from build123d import *

# Parameters (mm, degrees)
SKETCH2_R           = 47.5
SKETCH2_R_2         = 5
BOSS_EXTRUDE2_DEPTH = 26
CUT_EXTRUDE1_DEPTH  = 26


with BuildPart() as part:
    # Sketch2 → Boss-Extrude2 (new body)
    with BuildSketch(Plane.XY):
        with BuildLine():
            Line((-44.361418341, 36.582981874), (25.749824557, 121.601589362))
            ThreePointArc((25.749824557, 121.601589362), (35.699764064, 124.986391522), (43.181062365, 117.604768557))
            Line((43.181062365, 117.604768557), (70.382008245, 5.874854744))
            ThreePointArc((70.382008245, 5.874854744), (71.516417726, -3.340902868), (70.495441136, -12.569915818))
            Line((70.495441136, -12.569915818), (43.209420588, -130.966785703))
            ThreePointArc((43.209420588, -130.966785703), (35.417472002, -138.528541499), (25.323491774, -134.527769491))
            Line((25.323491774, -134.527769491), (-46.812831844, -33.388752219))
            ThreePointArc((-46.812831844, -33.388752219), (-57.464744559, 2.013239383), (-44.361418341, 36.582981874))
        make_face()
        with Locations(Location((0, 0, 0), (0, 0, 180))):
            Circle(SKETCH2_R, mode=Mode.SUBTRACT)
        with Locations(Location((33.464853834, 115.239331644, 0), (0, 0, 180))):
            Circle(SKETCH2_R_2, mode=Mode.SUBTRACT)
        with Locations(Location((33.464853834, -128.721029975, 0), (0, 0, 180))):
            Circle(SKETCH2_R_2, mode=Mode.SUBTRACT)
    extrude(amount=BOSS_EXTRUDE2_DEPTH)

    # Sketch3 → Cut-Extrude1 (cut)
    with BuildSketch(Plane(origin=(0, 0, 0), x_dir=(-1, 0, 0), z_dir=(0, 0, -1))):
        with BuildLine():
            Line((-33.26004361, 92.533263855), (-44.920341747, 51.273747369))
            ThreePointArc((-44.920341747, 51.273747369), (-44.16321834, 48.345074539), (-41.240708097, 47.564501493))
            Line((-41.240708097, 47.564501493), (2.410664417, 59.523781634))
            ThreePointArc((2.410664417, 59.523781634), (4.534059271, 61.712628945), (3.644196413, 64.629476961))
            Line((3.644196413, 64.629476961), (-28.346877964, 93.929713306))
            ThreePointArc((-28.346877964, 93.929713306), (-31.193307402, 94.603096407), (-33.26004361, 92.533263855))
        make_face()
        with BuildLine():
            Line((-41.486917876, -55.239236277), (2.503698589, -65.483626413))
            ThreePointArc((2.503698589, -65.483626413), (4.700165382, -67.55485567), (3.983155181, -70.48749158))
            Line((3.983155181, -70.48749158), (-28.256543188, -103.932412317))
            ThreePointArc((-28.256543188, -103.932412317), (-31.16488904, -104.755498955), (-33.313463379, -102.629569624))
            Line((-33.313463379, -102.629569624), (-45.064381475, -58.940258751))
            ThreePointArc((-45.064381475, -58.940258751), (-44.32436227, -56.076046257), (-41.486917876, -55.239236277))
        make_face()
    extrude(amount=-CUT_EXTRUDE1_DEPTH, mode=Mode.SUBTRACT)


solid = part.part
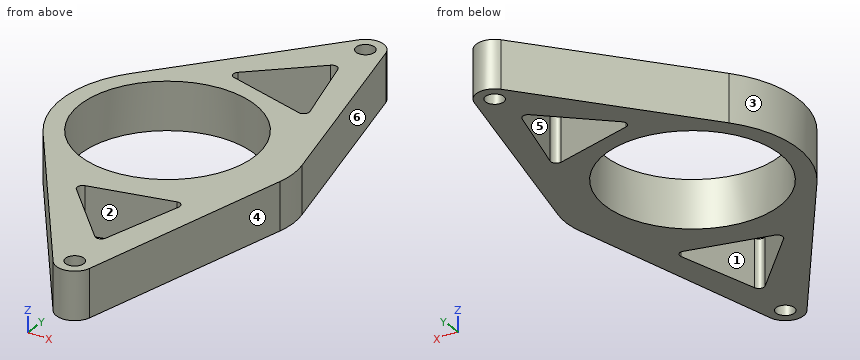
The listing builds one solid part. Answer for the finished solid, in the listing's coordinates (mm). Face numbers are marked on the shaded views. A direction names the side the tool comes from. Give positions to 0.01 mm unless a question says otherwise; leave off trailing zeros. Loops run counter-clockwise (first coordinate to the right, second up) from the corner with the lowest first, then second, coordinate; pieces in that order, holes last.
Item 1: Find the intervals of material crossed by line 1 along Y through (x, z) = (29, 19.5); line 2 along Y through (x, z) = (11, 24.75); line 3 along X through (y, z) = (88.5, 16), in increasing order.
Derived:
line 1: y = -137.67 to -130.97, -126.47 to -104.49, -58.15 to -37.62, 37.62 to 50.92, 94.38 to 112.99, 117.49 to 124.19
line 2: y = -114.45 to -86.03, -62.34 to -46.21, 46.21 to 55.85, 78.04 to 103.72
line 3: x = -1.55 to 22.42, 34.4 to 50.27
Item 2: Each of these flat-tipped pins is pushed along its axis until it touches: pin 1 Ø1 at (y, z) = (18.5, 18) entering from +X; pin 2 Ø8 at (y, z) = (-8, 12) entering from -X; pin 3 Ø2 at (x, z) = (-11.5, 20) entering from -Y. Where does it stop, or does it pass through?
Derived:
pin 1: stops at x = 67.43
pin 2: stops at x = -57.36
pin 3: stops at y = -84.3
Item 3: A cutting plane is placed at A-A (x = 12). Give the vertices of the cut face in (y, z), then the cut area to 3 significant figures.
Derived:
outline: (-115.85, 0) - (-87.07, 0) - (-87.07, 26) - (-115.85, 26) - close; (-62.11, 0) - (-45.96, 0) - (-45.96, 26) - (-62.11, 26) - close; (45.96, 0) - (55.58, 0) - (55.58, 26) - (45.96, 26) - close; (78.96, 0) - (104.93, 0) - (104.93, 26) - (78.96, 26) - close
area: 2,090 mm2
Item 4: Determine the mould class of the marked faces 1, 2, 3 and 4 for opening direction X: +X half, -X half, draft (parallel to the pull), parting line (faces both ways), or undercut.
Derived:
face 1: undercut
face 2: undercut
face 3: -X half
face 4: +X half
Item 5: A tool of negligible diameter and unlimited length cuts with its end or side. For the marked faces 5 and 6, from which of +Z, -Z, +X, -X, +Y, -Y can it reach the whole face along a straight path? Write none if from no direction.
Derived:
face 5: +Z, -Z
face 6: +Z, -Z, +X, +Y
Item 6: A cutting plane is placed at B-B (y = 90). Give the vertices of the cut face in (x, z), then the cut area to 3 significant figures.
Derived:
outline: (-0.31, 0) - (24.06, 0) - (24.06, 26) - (-0.31, 26) - close; (33.98, 0) - (49.9, 0) - (49.9, 26) - (33.98, 26) - close
area: 1,050 mm2
Item 7: A cutting plane is placed at C-C (x = -32). Give the vertices of the cut face in (y, z), then the cut area to 3 significant figures.
Derived:
outline: (-54.16, 0) - (-35.1, 0) - (-35.1, 26) - (-54.16, 26) - close; (35.1, 0) - (51.57, 0) - (51.57, 26) - (35.1, 26) - close
area: 924 mm2
Item 8: A cutting plane is placed at D-D (z = 19.5). Give the vertices of the cut face in (x, y), then the cut area to 3 significant figures.
Derived:
outline: (-46.81, -33.39) - (25.32, -134.53) arc R10 ccw to (43.21, -130.97) - (70.5, -12.57) arc R40 ccw to (70.38, 5.87) - (43.18, 117.6) arc R10 ccw to (25.75, 121.6) - (-44.36, 36.58) arc R57.5 ccw to start; hole circle Ø95 at (0, 0); hole (-3.98, -70.49) - (28.26, -103.93) arc R3 ccw to (33.31, -102.63) - (45.06, -58.94) arc R3 ccw to (41.49, -55.24) - (-2.5, -65.48) arc R3 ccw to start; hole (-3.64, 64.63) arc R3 ccw to (-2.41, 59.52) - (41.24, 47.56) arc R3 ccw to (44.92, 51.27) - (33.26, 92.53) arc R3 ccw to (28.35, 93.93) - close; hole circle Ø10 at (33.46, -128.72); hole circle Ø10 at (33.46, 115.24)
area: 10,600 mm2
